from build123d import *

# Parameters (mm, degrees)
BOSS_EXTRUDE1_DEPTH = 8
SKETCH2_R           = 1.1
CUT_EXTRUDE1_DEPTH  = 18.720045147
SKETCH3_R           = 1
CUT_EXTRUDE2_DEPTH  = 29.08914381
CUT_EXTRUDE3_DEPTH  = 2
FILLET1_R           = 2
FILLET2_R           = 1


with BuildPart() as part:
    # Sketch1 → Boss-Extrude1 (new body)
    with BuildSketch(Plane(origin=(0, 0, 0), x_dir=(1, 0, 0), z_dir=(0, 1, 0))):
        Polygon((-25, 1.25), (-25, 5), (0, 5), (0, -5), (-25, -5), (-25, -1.25), (-15, -1.25), (-15, 1.25), align=None)
    extrude(amount=BOSS_EXTRUDE1_DEPTH)

    # Sketch2 → Cut-Extrude1 (cut, through all)
    with BuildSketch(Plane.ZY.offset(15)):
        with Locations((0, 4)):
            Circle(SKETCH2_R)
    extrude(amount=-CUT_EXTRUDE1_DEPTH, mode=Mode.SUBTRACT)

    # Sketch3 → Cut-Extrude2 (cut, through all)
    with BuildSketch(Plane.XY.offset(5)):
        with Locations((-20, 4)):
            Circle(SKETCH3_R)
    extrude(amount=-CUT_EXTRUDE2_DEPTH, mode=Mode.SUBTRACT)

    # Sketch4 → Cut-Extrude3 (cut)
    with BuildSketch(Plane.XY.offset(5)):
        Polygon((-20, 1.546261356), (-17.875, 2.773130678), (-17.875, 5.226869322), (-20, 6.453738644), (-22.125, 5.226869322), (-22.125, 2.773130678), align=None)
    cut_extrude3 = extrude(amount=-CUT_EXTRUDE3_DEPTH, mode=Mode.SUBTRACT)

    # Mirror1: Cut-Extrude3 across plane
    add(cut_extrude3.mirror(Plane.XY), mode=Mode.SUBTRACT)

    # Fillet1
    fillet1_edges = [part.edges().sort_by_distance(p)[0] for p in [
        (0, 0, 0),
        (-15, 8, 0),
        (-25, 0, 3.125),
        (-20, 0, 1.25),
        (-15, 0, 0),
        (-20, 0, -1.25),
        (-20, 8, 1.25),
        (-25, 8, 3.125),
        (0, 8, 0),
        (-25, 8, -3.125),
        (-20, 8, -1.25),
        (-25, 0, -3.125),
    ]]
    fillet(fillet1_edges, radius=FILLET1_R)

    # Fillet2
    fillet2_edges = [part.edges().sort_by_distance(p)[0] for p in [
        (-25, 4, 5),
        (-12.5, 8, 5),
        (-12.5, 8, -5),
        (-12.5, 0, 5),
        (0, 4, 5),
        (-0.585786438, 7.414213562, 5),
        (-24.414213562, 0.585786438, 5),
        (-0.585786438, 0.585786438, 5),
        (-24.414213562, 7.414213562, 5),
        (-25, 4, -5),
        (-12.5, 0, -5),
        (0, 4, -5),
        (-0.585786438, 7.414213562, -5),
        (-24.414213562, 0.585786438, -5),
        (-0.585786438, 0.585786438, -5),
        (-24.414213562, 7.414213562, -5),
    ]]
    fillet(fillet2_edges, radius=FILLET2_R)


solid = part.part
Model file for the job. Use its own axes, mm. A direction names the side the tool comes from. Coordinates: 2 decimals unless noted, no trailing zeros. Write each loop counter-clockwise with the first axis right and the second up, starting at its lowest first coordinate (ties: lowest second). Pieces come first, ordered by that corner, then holes. Notation, with made-up numbers: (53.5, 64) -> (68.5, 64) arc R14 cw to (68.5, 90) -> close; hole circle Ø6 at (54, -2.75). An arc over 180 degrees is marked (long way). One line per item, written item: value. Start each with the question number.
1) Slice it at C-C on z = 3.75. Write the cut outline in (x, y) (3 decimals), then the cut area to 3 significant figures.
2) Flat gauge pins, fed straight in: pin 1 Ø3 at (x, y) = (-20, 4) entering from -Z; pin 2 Ø2.5 at (x, y) = (-20, 4) entering from +Z. Where does each tip first touch, or does it go through?
3) Which spindle directions (+Z, -Z, +X, -X, +Y, -Y) get a long thin tool onto all of the face, cutting with end or side? Do faces 1 (the face through (-14.13, 7.65, -0.05)), 2 (the face through (-21.08, 2.17, -4.01)), 3 (the face through (-18.92, 0.57, 1.85)). Say none if no direction does.
4) Slice it at D-D on y = 4.25. Count the separate pieces of the cut face and the enclosed holes in it, then the cut area to 3 significant figures.
5) Slice it at A-A on z = 0. Write the cut outline in (x, y), then the cut area to 3 significant figures.
6) Pull direction X, two halves, no side cores. Call faces 4 (the face through (-21.048, 5.849, 4.014)), 5 (the face through (-0.301, 3.972, 4.715)), 6 (the face through (-15, 3, 1)): +X half, -X half, draft (parallel to the pull), parting line (faces both ways), or undercut.
7) Slice it at B-B on x = -4.25. Write the cut outline in (y, z), then the cut area to 3 significant figures.
8) Probe probe 1 along Z at (x, y) = (-18, 4.25); probe 2 along Y at (x, z) = (-5.75, 0); probe 3 along X at (y, z) = (4.75, -3.75) (3 decimals). List the from-to ranges inside material, lowest first.
Answers follow:
1. outline: (-25, 2) arc R2 ccw to (-23, 0) -> (-2, 0) arc R2 ccw to (0, 2) -> (0, 6) arc R2 ccw to (-2, 8) -> (-23, 8) arc R2 ccw to (-25, 6) -> close; hole (-22.125, 2.773) -> (-20, 1.546) -> (-17.875, 2.773) -> (-17.875, 5.227) -> (-20, 6.454) -> (-22.125, 5.227) -> close
1. area: 181 mm2
2. pin 1: z = -3
2. pin 2: z = 3
3. face 1: -X, +Y
3. face 2: -Z
3. face 3: -X, -Y
4. separate pieces: 4
4. enclosed holes: 0
4. area: 168 mm2
5. outline: (-15, 2) arc R2 ccw to (-13, 0) -> (-2, 0) arc R2 ccw to (0, 2) -> (0, 2.9) -> (-15, 2.9) -> close; (-15, 5.1) -> (0, 5.1) -> (0, 6) arc R2 ccw to (-2, 8) -> (-13, 8) arc R2 ccw to (-15, 6) -> close
5. area: 83.6 mm2
6. face 4: undercut
6. face 5: +X half
6. face 6: -X half
7. outline: (0, -4) arc R1 ccw to (1, -5) -> (7, -5) arc R1 ccw to (8, -4) -> (8, 4) arc R1 ccw to (7, 5) -> (1, 5) arc R1 ccw to (0, 4) -> close; hole circle Ø2.2 at (4, 0)
7. area: 75.3 mm2
8. probe 1: -3 to -1.25, 1.25 to 3
8. probe 2: 0 to 2.9, 5.1 to 8
8. probe 3: -25 to -22.125, -17.875 to 0
